```python
from build123d import *

# Parameters (mm, degrees)
SKETCH1_R           = 90
SKETCH1_R_2         = 3.25
BOSS_EXTRUDE1_DEPTH = 3
SKETCH2_R           = 2.5
CUT_EXTRUDE1_DEPTH  = 3


with BuildPart() as part:
    # Sketch1 → Boss-Extrude1 (new body)
    with BuildSketch(Plane(origin=(0, 0, 0), x_dir=(1, 0, 0), z_dir=(0, 1, 0))):
        with Locations(Location((0, 0, 0), (0, 0, 270))):
            Circle(SKETCH1_R)
        with Locations(Location((37, 0, 0), (0, 0, 270))):
            Circle(SKETCH1_R_2, mode=Mode.SUBTRACT)
        with Locations(Location((11.433628792, -35.189091103, 0), (0, 0, 270))):
            Circle(SKETCH1_R_2, mode=Mode.SUBTRACT)
        with Locations(Location((-29.933628792, -21.748054335, 0), (0, 0, 270))):
            Circle(SKETCH1_R_2, mode=Mode.SUBTRACT)
        with Locations(Location((-29.933628792, 21.748054335, 0), (0, 0, 270))):
            Circle(SKETCH1_R_2, mode=Mode.SUBTRACT)
        with Locations(Location((11.433628792, 35.189091103, 0), (0, 0, 270))):
            Circle(SKETCH1_R_2, mode=Mode.SUBTRACT)
        with BuildLine():
            ThreePointArc((-32.941714384, 16.847654242), (-37, 0), (-32.941714384, -16.847654242))
            ThreePointArc((-32.941714384, -16.847654242), (-25.281781074, -18.368289134), (-26.202620919, -26.123220647))
            ThreePointArc((-26.202620919, -26.123220647), (-11.194944129, -35.265751459), (6.338065362, -36.453105869))
            ThreePointArc((6.338065362, -36.453105869), (9.811289571, -30.196044392), (16.298995441, -33.216603493))
            ThreePointArc((16.298995441, -33.216603493), (29.78558867, -21.95036919), (36.553209459, -5.732615303))
            ThreePointArc((36.553209459, -5.732615303), (31.25, 0), (36.553209459, 5.732615303))
            ThreePointArc((36.553209459, 5.732615303), (29.933628792, 21.748054335), (16.747604061, 32.992692497))
            ThreePointArc((16.747604061, 32.992692497), (9.656781074, 29.720516134), (5.843521783, 36.535643599))
            ThreePointArc((5.843521783, 36.535643599), (-11.433628792, 35.189091103), (-26.202620919, 26.123220647))
            ThreePointArc((-26.202620919, 26.123220647), (-25.281781074, 18.368289134), (-32.941714384, 16.847654242))
        make_face(mode=Mode.SUBTRACT)
    extrude(amount=BOSS_EXTRUDE1_DEPTH)

    # Sketch2 → Cut-Extrude1 (cut)
    with BuildSketch(Plane(origin=(0, 3, 0), x_dir=(1, 0, 0), z_dir=(0, 1, 0))):
        with Locations(Location((70, 0, 0), (0, 0, 270))):
            Circle(SKETCH2_R)
        with Locations(Location((48.244210623, 13.133778641, 0), (0, 0, 270))):
            Circle(SKETCH2_R)
        with Locations(Location((68.806307277, 29.844464796, 0), (0, 0, 270))):
            Circle(SKETCH2_R)
        with Locations(Location((73.207608177, -16.298653474, 0), (0, 0, 270))):
            Circle(SKETCH2_R)
        with Locations(Location((46.750227666, -17.731785391, 0), (0, 0, 270))):
            Circle(SKETCH2_R)
        with Locations(Location((56.631189606, -41.14496766, 0), (0, 0, 270))):
            Circle(SKETCH2_R)
        with Locations(Location((49.646090988, -56.216240088, 0), (0, 0, 270))):
            Circle(SKETCH2_R)
        with Locations(Location((27.399246723, -41.824410086, 0), (0, 0, 270))):
            Circle(SKETCH2_R)
        with Locations(Location((21.631189606, -66.573956141, 0), (0, 0, 270))):
            Circle(SKETCH2_R)
        with Locations(Location((7.121454451, -74.661133708, 0), (0, 0, 270))):
            Circle(SKETCH2_R)
        with Locations(Location((-2.417315202, -49.941531687, 0), (0, 0, 270))):
            Circle(SKETCH2_R)
        with Locations(Location((-21.631189606, -66.573956141, 0), (0, 0, 270))):
            Circle(SKETCH2_R)
        with Locations(Location((-38.123335637, -64.58801189, 0), (0, 0, 270))):
            Circle(SKETCH2_R)
        with Locations(Location((-31.310544882, -38.982685634, 0), (0, 0, 270))):
            Circle(SKETCH2_R)
        with Locations(Location((-56.631189606, -41.14496766, 0), (0, 0, 270))):
            Circle(SKETCH2_R)
        with Locations(Location((-68.806307277, -29.844464796, 0), (0, 0, 270))):
            Circle(SKETCH2_R)
        with Locations(Location((-48.244210623, -13.133778641, 0), (0, 0, 270))):
            Circle(SKETCH2_R)
        with Locations(Location((-70, 0, 0), (0, 0, 270))):
            Circle(SKETCH2_R)
        with Locations(Location((-73.207608177, 16.298653474, 0), (0, 0, 270))):
            Circle(SKETCH2_R)
        with Locations(Location((-46.750227666, 17.731785391, 0), (0, 0, 270))):
            Circle(SKETCH2_R)
        with Locations(Location((-56.631189606, 41.14496766, 0), (0, 0, 270))):
            Circle(SKETCH2_R)
        with Locations(Location((-49.646090988, 56.216240088, 0), (0, 0, 270))):
            Circle(SKETCH2_R)
        with Locations(Location((-27.399246723, 41.824410086, 0), (0, 0, 270))):
            Circle(SKETCH2_R)
        with Locations(Location((-21.631189606, 66.573956141, 0), (0, 0, 270))):
            Circle(SKETCH2_R)
        with Locations(Location((-7.121454451, 74.661133708, 0), (0, 0, 270))):
            Circle(SKETCH2_R)
        with Locations(Location((2.417315202, 49.941531687, 0), (0, 0, 270))):
            Circle(SKETCH2_R)
        with Locations(Location((21.631189606, 66.573956141, 0), (0, 0, 270))):
            Circle(SKETCH2_R)
        with Locations(Location((38.123335637, 64.58801189, 0), (0, 0, 270))):
            Circle(SKETCH2_R)
        with Locations(Location((31.310544882, 38.982685634, 0), (0, 0, 270))):
            Circle(SKETCH2_R)
        with Locations(Location((56.631189606, 41.14496766, 0), (0, 0, 270))):
            Circle(SKETCH2_R)
    extrude(amount=-CUT_EXTRUDE1_DEPTH, mode=Mode.SUBTRACT)


solid = part.part
```
Source: CAD feature listing. Evaluate the final solid. Frame: model axes, mm. Round coordinates to 2 decimals unless told otherwise and drop trailing zeros. Loops run counter-clockwise (first coordinate to the right, second up) from the corner with the lowest first, then second, coordinate; pieces in that order, holes last. Notation, with made-up numbers: M 48.5,-34 L 70.5,-34 A22 cw 70.5,-19 Z; hole C 84.5,83 d7. An arc over 180 degrees is marked long. Put each result on its own line as item: value.
(1) First-contact query: pin 1 (3 mm diameter, centred on x = -70, z = 0, fed in from +Y). Flat tip, straight axial feed; report the tip coordinate or a pass-through.
Solutions:
pin 1: through
(2) Section B-B, the plane y = 1.25. State how many separate pieces and enclosed holes the cut face has, and give its area (3 significant figures).
Solutions:
separate pieces: 1
enclosed holes: 36
area: 20,600 mm²
(3) Pull-direction query (Z, two-part tool) for faces 1 (the face through (1, 3, 39)), 2 (the face through (-50.685, 1.521, 12.592)); classes: released by +Z, released by -Z, zero draft, split by the parting line, or undercut.
Solutions:
face 1: zero draft
face 2: undercut
(4) Ray query, line 1 (Z direction, x = 56, y = 1.3); line 2 (Z direction, x = 68, y = 1.75); line 3 (X direction, y = 0.5, z = 19.5). Return the intervals inside material, ascending. Write a range as [from, to].
Solutions:
line 1: [-70.46, -43.56], [-38.73, 38.73], [43.56, 70.46]
line 2: [-58.96, -32.21], [-27.48, -1.5], [1.5, 58.96]
line 3: [-87.86, -32.28], [-27.59, -24.64], [31.44, 44.98], [48.52, 87.86]
(5) Section A-A, the plane z = 0. Return loops of the section in (x, y), and give its area (3 significant figures).
Solutions:
outline: M -90,0 L -72.5,0 L -72.5,3 L -90,3 Z; M -67.5,0 L -37,0 L -37,3 L -67.5,3 Z; M 31.25,0 L 33.75,0 L 33.75,3 L 31.25,3 Z; M 40.25,0 L 67.5,0 L 67.5,3 L 40.25,3 Z; M 72.5,0 L 90,0 L 90,3 L 72.5,3 Z
area: 286 mm²
